Check sheet for the modelled part. Datum: model origin and axes. Units: mm. Face numbers are marked on the shaded views. A direction names the side the tool comes from. Round coordinates to 2 decimals unless told otherwise and drop trailing zeros. Write each loop counter-clockwise with the first axis right and the second up, starting at its lowest first coordinate (ties: lowest second). Pieces come first, ordered by that corner, then holes. Notation, with made-up numbers: (72, -1) -> (112, -1) arc R16 ccw to (112, 22) -> close; hole circle Ø7 at (-7, 30). An arc over 180 degrees is marked (long way). One line per item, written item: value.
from build123d import *

# Parameters (mm, degrees)
SKETCH1_W           = 90
SKETCH1_H           = 55
BOSS_EXTRUDE1_DEPTH = 30
SKETCH2_W           = 60
SKETCH2_H           = 40
CUT_EXTRUDE1_DEPTH  = 31
SKETCH3_R           = 2
CUT_EXTRUDE2_DEPTH  = 31
LPATTERN1_COUNT     = 3
LPATTERN1_PITCH     = 10
LPATTERN1_COL_COUNT = 3
LPATTERN1_COL_PITCH = 10
FILLET1_R           = 10
FILLET2_R           = 5


with BuildPart() as part:
    # Sketch1 → Boss-Extrude1 (new body)
    with BuildSketch(Plane.XY):
        Rectangle(SKETCH1_W, SKETCH1_H)
    extrude(amount=BOSS_EXTRUDE1_DEPTH)

    # Sketch2 → Cut-Extrude1 (cut, through all)
    with BuildSketch(Plane.XY.offset(30)):
        Rectangle(SKETCH2_W, SKETCH2_H)
    extrude(amount=-CUT_EXTRUDE1_DEPTH, mode=Mode.SUBTRACT)

    # Sketch3 → Cut-Extrude2 (cut, through all)
    with BuildSketch(Plane(origin=(0, 0, 0), x_dir=(-1, 0, 0), z_dir=(0, 0, -1))):
        with Locations((-37.5, 0)):
            Circle(SKETCH3_R)
        with Locations((37.5, 0)):
            Circle(SKETCH3_R)
    cut_extrude2 = extrude(amount=-CUT_EXTRUDE2_DEPTH, mode=Mode.SUBTRACT)

    # LPattern1: Cut-Extrude2 ×3
    with Locations(*[(0, -i * LPATTERN1_PITCH, 0) for i in range(1, LPATTERN1_COUNT)]):
        add(cut_extrude2, mode=Mode.SUBTRACT)

    # LPattern1 col: Cut-Extrude2 ×3
    with Locations(*[(0, i * LPATTERN1_COL_PITCH, 0) for i in range(1, LPATTERN1_COL_COUNT)]):
        add(cut_extrude2, mode=Mode.SUBTRACT)

    # Fillet1
    fillet1_edges = [part.edges().sort_by_distance(p)[0] for p in [
        (45, -27.5, 15),
        (-45, -27.5, 15),
        (-45, 27.5, 15),
        (45, 27.5, 15),
    ]]
    fillet(fillet1_edges, radius=FILLET1_R)

    # Fillet2
    fillet2_edges = [part.edges().sort_by_distance(p)[0] for p in [
        (30, 20, 15),
        (30, -20, 15),
        (-30, -20, 15),
        (-30, 20, 15),
    ]]
    fillet(fillet2_edges, radius=FILLET2_R)


solid = part.part
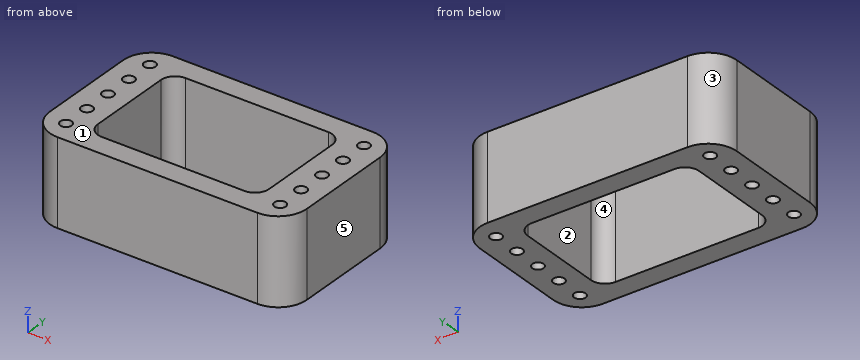
Item 1: Sectioned sample at A-A (x = 15.5). Enter the section's corners in (y, z), then the cut area to 3 significant figures.
Result set:
outline: (-27.5, 0) -> (-20, 0) -> (-20, 30) -> (-27.5, 30) -> close; (20, 0) -> (27.5, 0) -> (27.5, 30) -> (20, 30) -> close
area: 450 mm^2
Item 2: Material ranges on line 1 along Y through (x, z) = (14, 17.5); line 2 along X through (y, z) = (-13, 28.25); line 3 along Y through (x, z) = (-37.5, 20.5), recorded low to high.
Result set:
line 1: -27.5 to -20, 20 to 27.5
line 2: -45 to -30, 30 to 45
line 3: -27.18 to -22, -18 to -12, -8 to -2, 2 to 8, 12 to 18, 22 to 27.18
Item 3: Sectioned sample at D-D (y = 0). Enter the section's corners in (x, z), then the cut area to 3 significant figures.
Result set:
outline: (-45, 0) -> (-39.5, 0) -> (-39.5, 30) -> (-45, 30) -> close; (-35.5, 0) -> (-30, 0) -> (-30, 30) -> (-35.5, 30) -> close; (30, 0) -> (35.5, 0) -> (35.5, 30) -> (30, 30) -> close; (39.5, 0) -> (45, 0) -> (45, 30) -> (39.5, 30) -> close
area: 660 mm^2
Item 4: Sectioned sample at B-B (z = 10). State how many separate pieces and enclosed holes the cut face has, then the cut area to 3 significant figures.
Result set:
separate pieces: 1
enclosed holes: 11
area: 2,360 mm^2
Item 5: Depth check by flat-ended pin: pin 1 (3 mm diameter, centred on x = -37.5, y = 10, fed in from -Z); pin 2 (6 mm diameter, centred on x = 35.5, z = 6, fed in from +Y); pin 3 (5 mm diameter, centred on y = -21, z = 20, fed in from +X). Enter the tip coordinate at first touch or a pass-through.
Result set:
pin 1: through
pin 2: y = 27.5
pin 3: x = 44.95
Item 6: Sectioned sample at C-C (y = 13.5). Enter the section's corners in (x, z).
Result set:
outline: (-45, 0) -> (-30, 0) -> (-30, 30) -> (-45, 30) -> close; (30, 0) -> (45, 0) -> (45, 30) -> (30, 30) -> close
Item 7: Release check for a two-part mould opening along Y. For the marked faces 1, 2 and 3 record: pulls with the +Y half, pulls with the -Y half, needs draft (parallel to the pull), parting line crosses it, or undercut.
Result set:
face 1: needs draft
face 2: undercut
face 3: pulls with the +Y half
Item 8: Tool access check on the marked faces 4 and 5. Record the directions out of +Z, -Z, +X, -X, +Y, -Y that give a thin tool (end or side, any length) a straight path to the whole face; none if there is none.
Result set:
face 4: +Z, -Z
face 5: +Z, -Z, +X, +Y, -Y
